Verification items for the finished model (mm, model axes). Coordinates: 2 decimals unless noted, no trailing zeros. Order: outer loops, then holes, each group sorted by start corner. A loop starts at its lowest first (then second) coordinate and runs counter-clockwise, first axis right, second up.
Q1. Cross-section at C-C, the plane x = 114.3. Record the boundary of the cut face in (y, z) (3 decimals), and give its area (3 significant figures).
Q2. Draft check along X on faces 1 (the cylindrical face through (151.42, 47.68, 0.4)), 2 (the cylindrical face through (-136.504, 0.977, -0.4)), 3 (the flat face through (-2, 2, 28.575)). Enter one of: pulls with the +X half, pulls with the -X half, needs draft (parallel to the pull), parting line crosses it, or undercut.
Q3. Depth check by flat-ended pin: P1, Ø6, axis at x = -76.5, z = -5.5, coming from the +Y side; P2, Ø8, axis at y = 96, z = -5.5, coming from the -X side; P3, Ø10, axis at y = 15, z = -5.5, coming from the +X side; P4, Ø8, axis at x = 119, y = -111.5, coming from the +Z side. Enter the tip coordinate at first touch or a pass-through.
Q4. Cross-section at A-A, the plane y = 0. Record the boundary of the cut face in (x, z) (3 decimals).
Q5. Cross-section at B-B, the plane x = 70.5. Record the boundary of the cut face in (y, z) (3 decimals), and give its area (3 significant figures).
Q6. Thickness scan on line 1 (Y direction, x = -57.15, z = 11.5); line 2 (X direction, y = -79, z = 7); line 3 (X direction, y = 103.5, z = -22). Record the ranges inside material, lowest first.
Q7. Cross-section at D-D, the plane z = 12. Record the boundary of the cut face in (x, y) (3 decimals), and give its area (3 significant figures).
from build123d import *

# Parameters (mm, degrees)
SKETCH1_R           = 158.75
SKETCH1_R_2         = 22.225
BOSS_EXTRUDE1_DEPTH = 28.575


with BuildPart() as part:
    # Sketch1 → Boss-Extrude1 (new, symmetric)
    with BuildSketch(Plane(origin=(0, 0, 0), x_dir=(0, 1, 0), z_dir=(0, 0, 1))):
        with Locations(Location((0, 0, 0), (0, 0, 270))):
            Circle(SKETCH1_R)
        with Locations(Location((0, 114.3, 0), (0, 0, 270))):
            Circle(SKETCH1_R_2, mode=Mode.SUBTRACT)
        with Locations(Location((98.986703653, 57.15, 0), (0, 0, 270))):
            Circle(SKETCH1_R_2, mode=Mode.SUBTRACT)
        with Locations(Location((98.986703653, -57.15, 0), (0, 0, 270))):
            Circle(SKETCH1_R_2, mode=Mode.SUBTRACT)
        with Locations(Location((0, -114.3, 0), (0, 0, 270))):
            Circle(SKETCH1_R_2, mode=Mode.SUBTRACT)
        with Locations(Location((-98.986703653, -57.15, 0), (0, 0, 270))):
            Circle(SKETCH1_R_2, mode=Mode.SUBTRACT)
        with Locations(Location((-98.986703653, 57.15, 0), (0, 0, 270))):
            Circle(SKETCH1_R_2, mode=Mode.SUBTRACT)
    extrude(amount=BOSS_EXTRUDE1_DEPTH, both=True)


solid = part.part
Check values:
1. outline: (-110.168, -28.575) - (-22.225, -28.575) - (-22.225, 28.575) - (-110.168, 28.575) - close; (22.225, -28.575) - (110.168, -28.575) - (110.168, 28.575) - (22.225, 28.575) - close
1. area: 10,100 mm2
2. face 1: parting line crosses it
2. face 2: undercut
2. face 3: needs draft
3. P1: stops at y = 140.71
3. P2: stops at x = -129.37
3. P3: stops at x = 158.43
3. P4: passes through
4. outline: (-158.75, -28.575) - (-136.525, -28.575) - (-136.525, 28.575) - (-158.75, 28.575) - close; (-92.075, -28.575) - (92.075, -28.575) - (92.075, 28.575) - (-92.075, 28.575) - close; (136.525, -28.575) - (158.75, -28.575) - (158.75, 28.575) - (136.525, 28.575) - close
5. outline: (-142.237, -28.575) - (-116.755, -28.575) - (-116.755, 28.575) - (-142.237, 28.575) - close; (-81.218, -28.575) - (81.218, -28.575) - (81.218, 28.575) - (-81.218, 28.575) - close; (116.755, -28.575) - (142.237, -28.575) - (142.237, 28.575) - (116.755, 28.575) - close
5. area: 12,200 mm2
6. line 1: y = -148.11 to -121.21, -76.76 to 76.76, 121.21 to 148.11
6. line 2: x = -137.7 to -66.87, -47.43 to 47.43, 66.87 to 137.7
6. line 3: x = -120.37 to -78.91, -35.39 to 35.39, 78.91 to 120.37
7. outline: circle Ø317.5 at (0, 0); hole circle Ø44.45 at (-114.3, 0); hole circle Ø44.45 at (-57.15, -98.987); hole circle Ø44.45 at (-57.15, 98.987); hole circle Ø44.45 at (57.15, -98.987); hole circle Ø44.45 at (57.15, 98.987); hole circle Ø44.45 at (114.3, 0)
7. area: 69,900 mm2
